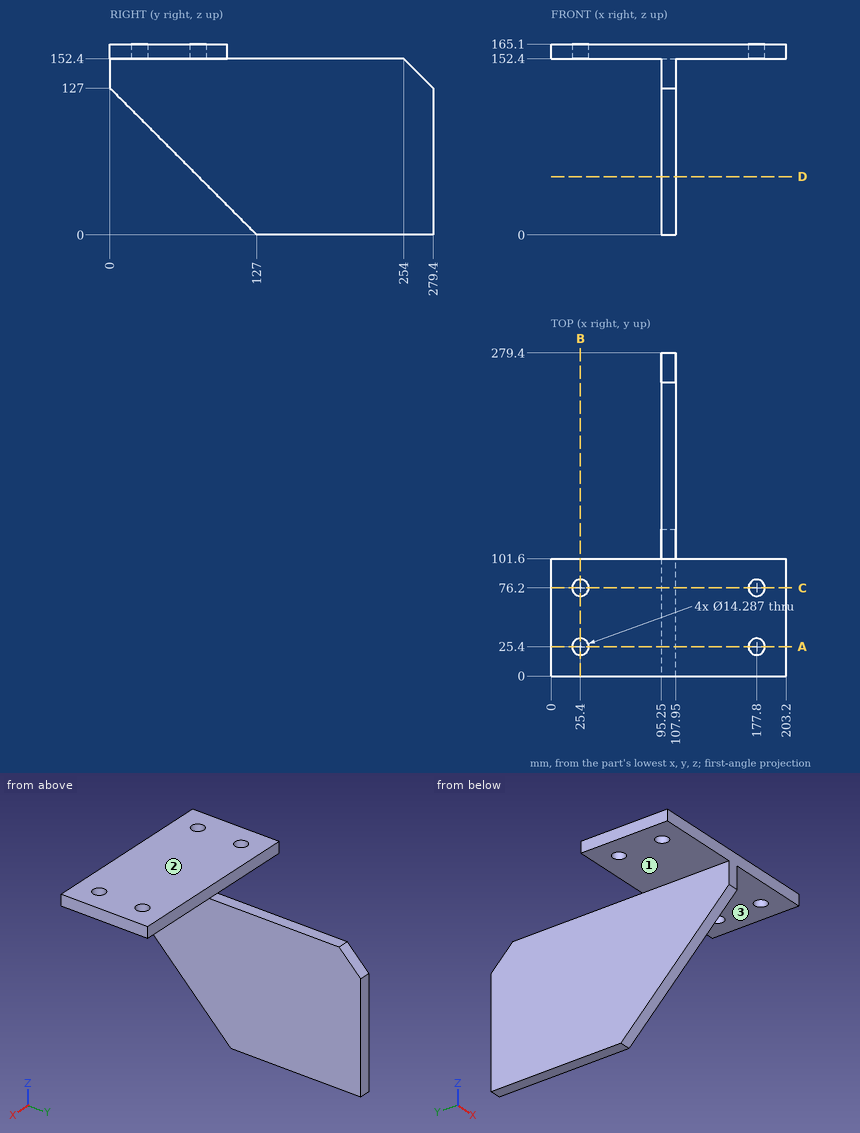
Can you work these out from the drawing? Everything is in mm from the part's minimum corner. A direction names the side the tool comes from. Give positions to 0.01 mm unless a question says otherwise; leave off trailing zeros. Loops run counter-clockwise (first coordinate to the right, second up) from the corner with the lowest first, then second, coordinate; pieces in that order, holes last. Notation, with made-up numbers: M 26,72 L 80,72 A34 ccw 80,106 Z; hole C 28.5,60 d4. An arc over 180 degrees is marked long. Put each result on its own line as item: value. Start each with the question number.
(1) I want a section at B-B on x = 25.4. Please give me the cut outline in (y, z).
(2) I want a section at A-A on y = 25.4. Please give me the cut outline in (x, z), then the cut area to 3 significant figures.
(3) For the marked faces 1, 2 and 3, which set-ups out of +Z, -Z, +X, -X, +Y, -Y let a thin tool reach every point of the face, with its end or its side?
(4) Will these pins go through, and if not, where does the flat tip stop? pin 1 Ø3 at (y, z) = (130, 70) entering from +X; pin 2 Ø10 at (x, z) = (67, 155.5) entering from +Y; pin 3 Ø1.5 at (y, z) = (209, 61.5) entering from -X; pin 4 Ø13 at (x, y) = (177.8, 25.4) entering from +Z.
(5) I want a section at D-D on z = 50.5. Please give me the cut outline in (x, y), then the cut area to 3 significant figures.
(6) I need wall thicknesses on line 1 along Y through (x, z) = (177.8, 159.5); line 2 along X through (y, z) = (76, 161); line 3 along X through (y, z) = (238, 89). Which ranges of each line are inside material? Lowest first, please. Write a range as [from, to].
(7) I want a section at C-C on y = 76.2. Please give me the cut outline in (x, z), then the cut area to 3 significant figures.
Answer block:
1. outline: M 0,152.4 L 18.26,152.4 L 18.26,165.1 L 0,165.1 Z; M 32.54,152.4 L 69.06,152.4 L 69.06,165.1 L 32.54,165.1 Z; M 83.34,152.4 L 101.6,152.4 L 101.6,165.1 L 83.34,165.1 Z
2. outline: M 0,152.4 L 18.26,152.4 L 18.26,165.1 L 0,165.1 Z; M 32.54,152.4 L 95.25,152.4 L 95.25,101.6 L 107.95,101.6 L 107.95,152.4 L 170.66,152.4 L 170.66,165.1 L 32.54,165.1 Z; M 184.94,152.4 L 203.2,152.4 L 203.2,165.1 L 184.94,165.1 Z
2. area: 2,860 mm^2
3. face 1: -Z, -X, +Y, -Y
3. face 2: +Z, +X, -X, +Y, -Y
3. face 3: -Z, +X, +Y, -Y
4. pin 1: x = 107.95
4. pin 2: y = 101.6
4. pin 3: x = 95.25
4. pin 4: through
5. outline: M 95.25,76.5 L 107.95,76.5 L 107.95,279.4 L 95.25,279.4 Z
5. area: 2,580 mm^2
6. line 1: [0, 18.26], [32.54, 69.06], [83.34, 101.6]
6. line 2: [0, 18.26], [32.54, 170.66], [184.94, 203.2]
6. line 3: [95.25, 107.95]
7. outline: M 0,152.4 L 18.26,152.4 L 18.26,165.1 L 0,165.1 Z; M 32.54,152.4 L 95.25,152.4 L 95.25,50.8 L 107.95,50.8 L 107.95,152.4 L 170.66,152.4 L 170.66,165.1 L 32.54,165.1 Z; M 184.94,152.4 L 203.2,152.4 L 203.2,165.1 L 184.94,165.1 Z
7. area: 3,510 mm^2
